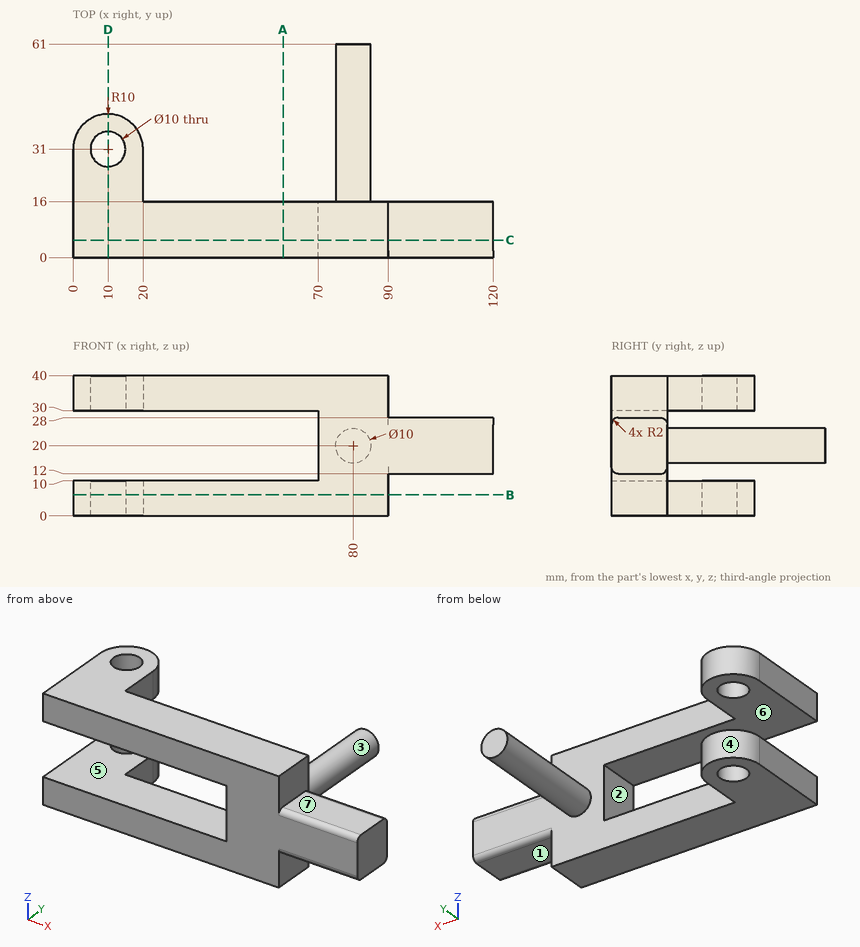
For this review, use the dimensioned drawing (mm, ordinates from the lowest corner) and the shaded views. A direction names the side the tool comes from. Coordinates: 2 decimals unless noted, no trailing zeros. Loops run counter-clockwise (first coordinate to the right, second up) from the corner with the lowest first, then second, coordinate; pieces in that order, holes last. Notation, with made-up numbers: (27.5, 25.5) -> (38.5, 25.5) arc R27 ccw to (38.5, 61.5) -> close; hole circle Ø7 at (33.25, 6). An arc over 180 degrees is marked (long way). Use a Markdown table: item, result. Add a question column.
1. Machinability: for the marked faces 1, 2 and 3, which of the approach directions +Z, -Z, +X, -X, +Y, -Y give a long, thin tool a straight path to every point of the face, cutting with its end or side? Answer none if there is none.
2. Add section B-B on z = 6. Write out the cut boundary in (x, y).
3. To check wall thickness, follow line 1 (Y direction, x = 10, z = 6); line 2 (Z direction, x = 8.5, y = 6); line 3 (Y direction, x = 54.5, z = 7.5). State the ranges of each line that lie inside material, in increasing order.
4. Add section C-C on y = 5. Write out the cut boundary in (x, z).
5. Add section A-A on x = 60. Write out the cut boundary in (y, z).
6. Draft analysis for pull direction Z (two halves, no side actions). For the marked faces 4, 5, 6 and 7, state which applies: pulls with the +Z half, pulls with the -Z half, needs draft (parallel to the pull), parting line crosses it, or undercut.
7. Clearance check with flat-ended pins moving along their axes: pin 1 Ø7 at (y, z) = (11.5, 32) entering from +X; pin 2 Ø17.5 at (y, z) = (9, 21) entering from -X; pin 3 Ø8 at (y, z) = (27, 3.5) entering from +X; pin 4 Ø10 at (y, z) = (49, 8) entering from -X. State where each tip first meets the part, or that it passes through.
8. Add section D-D on x = 10. Write out the cut boundary in (y, z).
Returned:
| question | item | result |
|---|---|---|
| 1 | face 1 | -Z, +X, +Y, -Y |
| 1 | face 2 | -X, +Y, -Y |
| 1 | face 3 | +Y |
| 2 | outline | (0, 0) -> (90, 0) -> (90, 16) -> (20, 16) -> (20, 31) arc R10 ccw to (0, 31) -> close; hole circle Ø10 at (10, 31) |
| 3 | line 1 | y = 0 to 26, 36 to 41 |
| 3 | line 2 | z = 0 to 10, 30 to 40 |
| 3 | line 3 | y = 0 to 16 |
| 4 | outline | (0, 0) -> (90, 0) -> (90, 12) -> (120, 12) -> (120, 28) -> (90, 28) -> (90, 40) -> (0, 40) -> (0, 30) -> (70, 30) -> (70, 10) -> (0, 10) -> close |
| 5 | outline | (0, 0) -> (16, 0) -> (16, 10) -> (0, 10) -> close; (0, 30) -> (16, 30) -> (16, 40) -> (0, 40) -> close |
| 6 | face 4 | needs draft |
| 6 | face 5 | undercut |
| 6 | face 6 | undercut |
| 6 | face 7 | pulls with the +Z half |
| 7 | pin 1 | stops at x = 90 |
| 7 | pin 2 | stops at x = 70 |
| 7 | pin 3 | stops at x = 20 |
| 7 | pin 4 | passes through |
| 8 | outline | (0, 0) -> (26, 0) -> (26, 10) -> (0, 10) -> close; (0, 30) -> (26, 30) -> (26, 40) -> (0, 40) -> close; (36, 0) -> (41, 0) -> (41, 10) -> (36, 10) -> close; (36, 30) -> (41, 30) -> (41, 40) -> (36, 40) -> close |
